Part print with two shaded views. Sizes in mm from the minimum x, y, z corner. A direction names the side the tool comes from. Coordinates: 2 decimals unless noted, no trailing zeros. Loops run counter-clockwise (first coordinate to the right, second up) from the corner with the lowest first, then second, coordinate; pieces in that order, holes last. Notation, with made-up numbers: (29.25, 58.5) -> (72.25, 58.5) arc R21 ccw to (72.25, 94.5) -> close; hole circle Ø11 at (23.5, -15). An arc over 180 degrees is marked (long way). Return JSON: item names as keys, results as strings. Group by question number.
(1) Saw through at C-C on y = 10. Write the cut outline in (x, z), then the cut area to 3 significant figures.
(2) Probe L1, parallel to Y at x = 8, z = 53; L2, parallel to Z at x = 9, y = 4.25; L3, parallel to Z at x = 11.5, y = 13. List the from-to ranges inside material, lowest first.
(3) Saw through at A-A on x = 69. Write the cut outline in (y, z), then the cut area to 3 significant figures.
(4) Tool access for the marked faces 1 and 2: list every direction of +Z, -Z, +X, -X, +Y, -Y with a clear straight run to the whole face (end or side of a thin tool).
(5) Flat gauge pins, fed straight in: pin 1 Ø6 at (x, z) = (29.5, 35) entering from +Y; pin 2 Ø5 at (y, z) = (16, 37.5) entering from -X; pin 3 Ø1.6 at (x, z) = (69, 35) entering from +Y. Where does each tip first touch, or does it go through?
(6) Saw through at D-D on z = 8.5. Write the cut outline in (x, y), then the cut area to 3 significant figures.
(7) Saw through at B-B on x = 10. Write the cut outline in (y, z), then the cut area to 3 significant figures.
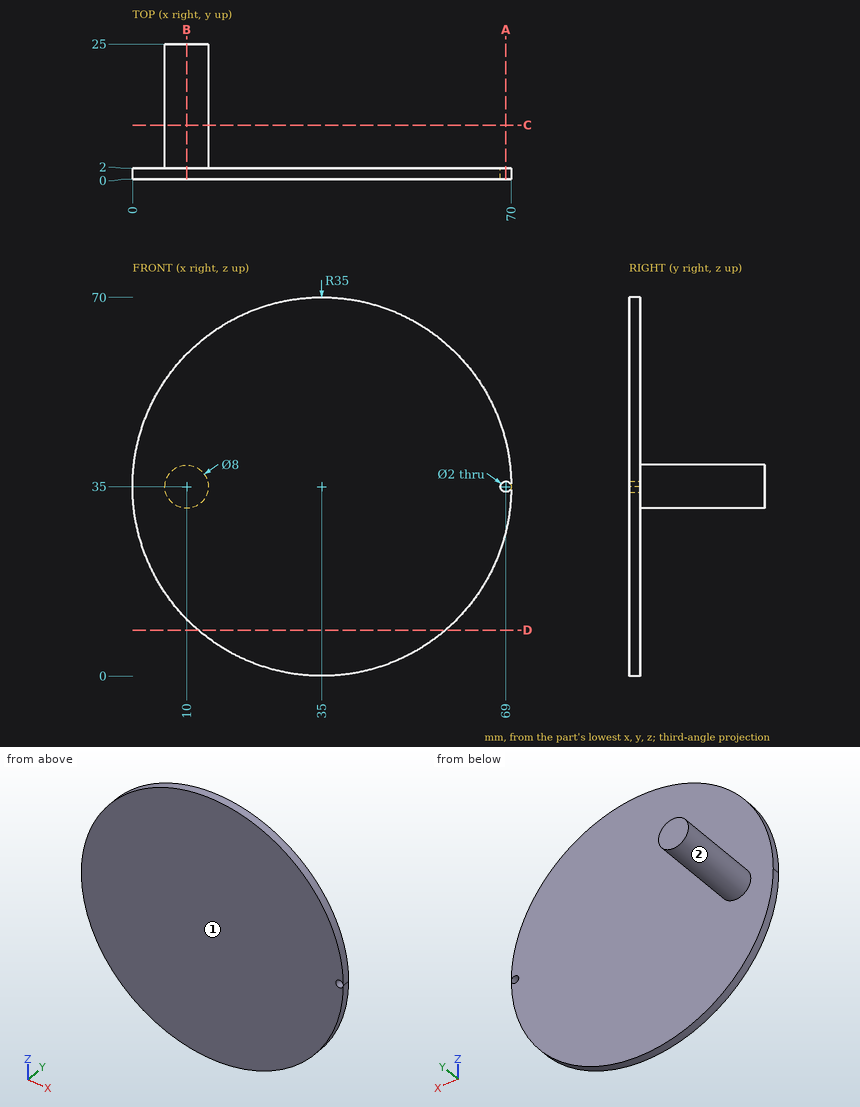
Geometry results:
{
 "1": {"outline": "circle Ø8 at (10, 35)", "area": "50.3 mm²"},
 "2": {"L1": "0 to 2", "L2": "31.13 to 38.87", "L3": "31.29 to 38.71"},
 "3": {"outline": "(0, 26.69) -> (2, 26.69) -> (2, 34) -> (0, 34) -> close; (0, 36) -> (2, 36) -> (2, 43.31) -> (0, 43.31) -> close", "area": "29.2 mm²"},
 "4": {"face 1": "+Z, -Z, +X, -X, -Y", "face 2": "+Y"},
 "5": {"pin 1": "y = 2", "pin 2": "x = 6", "pin 3": "through"},
 "6": {"outline": "(12.14, 0) -> (57.86, 0) -> (57.86, 2) -> (12.14, 2) -> close", "area": "91.5 mm²"},
 "7": {"outline": "(0, 10.51) -> (2, 10.51) -> (2, 31) -> (25, 31) -> (25, 39) -> (2, 39) -> (2, 59.49) -> (0, 59.49) -> close", "area": "282 mm²"}
}
